Input: dimensioned drawing with shaded views. Units: mm. Origin: part minimum x, y, z. Round coordinates to 2 decimals unless told otherwise and drop trailing zeros. Write each loop counter-clockwise with the first axis right and the second up, starting at its lowest first coordinate (ties: lowest second). Pieces come first, ordered by that corner, then holes. Notation, with made-up numbers: M -24,-6 L 14,-6 A16 ccw 14,23 Z; hole C 47,36.25 d8. An arc over 180 degrees is marked long. Answer in a Markdown table with one row per item. Add a question column.
Item 1: Cut plane A-A on z = 2.75. Return loops of the section in (x, y), and give its area (4 significant figures).
Item 2: Contact query for a flat-ended pin moving along its axis: pin 1 (1.2 mm diameter, centred on y = 168.5, z = 2.5, fed in from -X). Output: stop coordinate, or through.
Item 3: Material intervals for probe 1 along Y at (x, z) = (14.5, 2.35); probe 2 along X at (y, z) = (128.5, 1.2), sorted ascending.
Item 4: Cut plane B-B on y = 159.5. Return loops of the section in (x, z).
Item 5: Cut plane C-C on x = 15. Return loops of the section in (y, z), and give its area (3 significant figures).
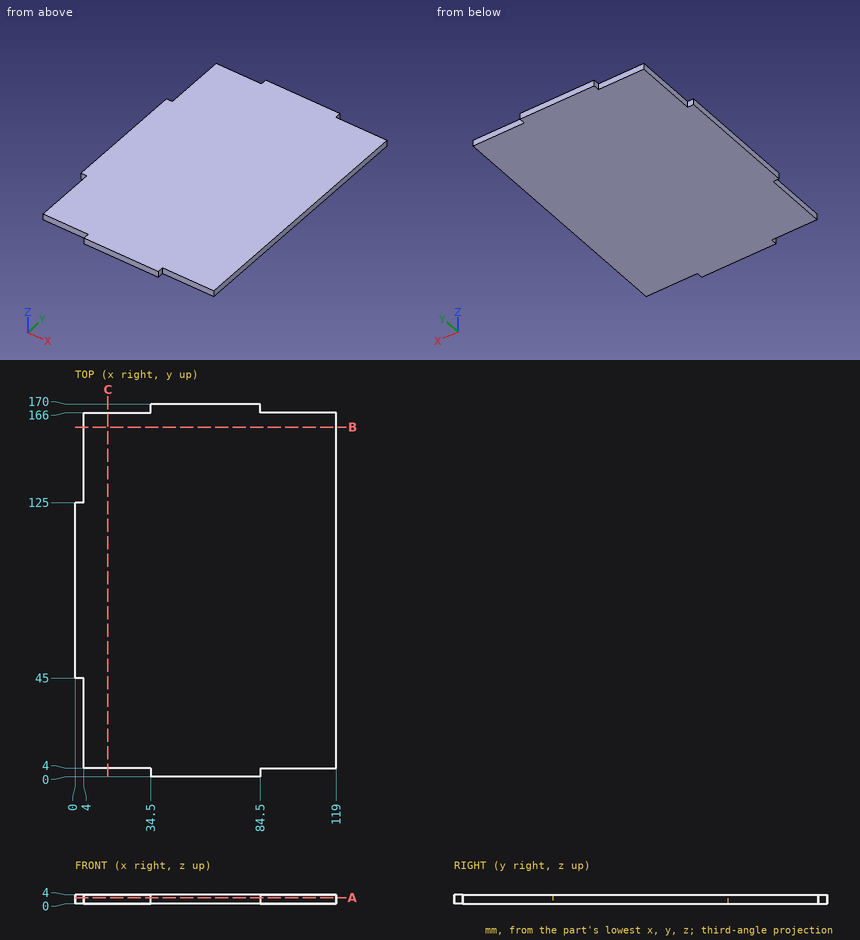
Results below:
| question | item | result |
|---|---|---|
| 1 | outline | M 0,45 L 4,45 L 4,4 L 34.5,4 L 34.5,0 L 84.5,0 L 84.5,4 L 119,4 L 119,166 L 84.5,166 L 84.5,170 L 34.5,170 L 34.5,166 L 4,166 L 4,125 L 0,125 Z |
| 1 | area | 19,350 mm2 |
| 2 | pin 1 | x = 34.5 |
| 3 | probe 1 | 4 to 166 |
| 3 | probe 2 | 4 to 119 |
| 4 | outline | M 4,0 L 119,0 L 119,4 L 4,4 Z |
| 5 | outline | M 4,0 L 166,0 L 166,4 L 4,4 Z |
| 5 | area | 648 mm2 |
